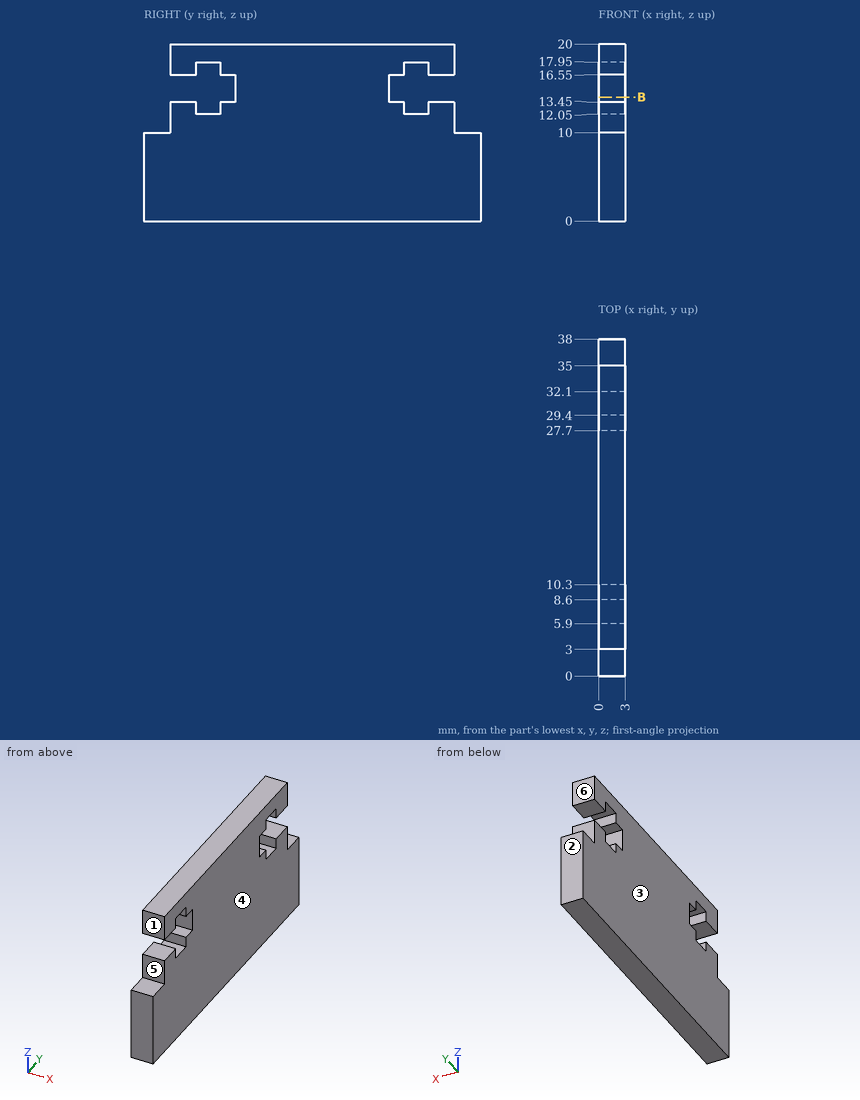
Geometry check sheet. Reference: drawing and pictorial views, mm from the part's lowest x, y, z. A direction names the side the tool comes from. Round coordinates to 2 decimals unless told otherwise and drop trailing zeros. Loops run counter-clockwise (first coordinate to the right, second up) from the corner with the lowest first, then second, coordinate; pieces in that order, holes last. Notation, with made-up numbers: M -31,-31.75 L -23,-31.75 A14 ccw -23,-12.75 Z; hole C 15.25,24 d7. An arc over 180 degrees is marked long. Return JSON: item names as keys, results as strings. Group by question number.
(1) Set-up check for the marked faces 4, 5 and 6: record each of +Z, -Z, +X, -X, +Y, -Y from which the full face is reachable in a straight line by a thin tool's end or side.
(2) Go/stop test with flat-tipped pins: pin 1 (0.9 mm diameter, centred on x = 2, z = 12, fed in from +Y); pin 2 (1.5 mm diameter, centred on x = 1.5, z = 13, fed in from -Y); pin 3 (0.9 mm diameter, centred on x = 1, y = 1.5, fed in from +Z). Record where each tip stops, or that it passes through.
(3) Mould release check, pull along Y, two halves, no side actions. Record for the marked faces 1, 2 and 3: pulls with the +Y half, pulls with the -Y half, needs draft (parallel to the pull), parting line crosses it, or undercut.
(4) Scan lines: line 1 along Y through (x, z) = (0.8, 17.25); line 2 along Z through (x, y) = (0.35, 34); line 3 along Z through (x, y) = (0.55, 6.5). Record each from-to range of solid material in increasing order. Write a range as [from, to].
(5) Section check B-B, the plane z = 14. Enter the section's corners in (x, y), and give its area (3 significant figures).
Data:
{
 "1": {"face 4": "+Z, -Z, +X, +Y, -Y", "face 5": "+Z, +X, -X, -Y", "face 6": "+Z, +X, -X, +Y"},
 "2": {"pin 1": "y = 35", "pin 2": "y = 3", "pin 3": "z = 10"},
 "3": {"face 1": "pulls with the -Y half", "face 2": "pulls with the +Y half", "face 3": "needs draft"},
 "4": {"line 1": "[3, 5.9], [8.6, 29.4], [32.1, 35]", "line 2": "[0, 13.45], [16.55, 20]", "line 3": "[0, 12.05], [17.95, 20]"},
 "5": {"outline": "M 0,10.3 L 3,10.3 L 3,27.7 L 0,27.7 Z", "area": "52.2 mm²"}
}
